```python
from build123d import *

# Parameters (mm, degrees)
BOSS_EXTRUDE1_DEPTH = 40
SKETCH2_R           = 27
CUT_EXTRUDE3_DEPTH  = 10
SKETCH4_R           = 19
CUT_EXTRUDE4_DEPTH  = 10
SKETCH5_R           = 19
BOSS_EXTRUDE2_DEPTH = 20
SKETCH6_R           = 10
CUT_EXTRUDE6_DEPTH  = 20
BOSS_EXTRUDE4_START = 64
SKETCH7_R           = 5
BOSS_EXTRUDE4_DEPTH = 10


with BuildPart() as part:
    # Sketch1 → Boss-Extrude1 (new body)
    with BuildSketch(Plane.XY):
        Polygon((0, 0), (0, 64), (-6, 64), (-6, 69), (3, 100), (73, 100), (82, 69), (82, 64), (76, 64), (76, 0), (56, 0), (56, 20), (20, 20), (20, 0), align=None)
    extrude(amount=BOSS_EXTRUDE1_DEPTH)

    # Sketch2 → Cut-Extrude3 (cut)
    with BuildSketch(Plane.XY.offset(40)):
        with Locations((38, 100)):
            Circle(SKETCH2_R)
    extrude(amount=-CUT_EXTRUDE3_DEPTH, mode=Mode.SUBTRACT)

    # Sketch4 → Cut-Extrude4 (cut)
    with BuildSketch(Plane.XY.offset(30)):
        with Locations((38, 100)):
            Circle(SKETCH4_R)
    extrude(amount=-CUT_EXTRUDE4_DEPTH, mode=Mode.SUBTRACT)

    # Sketch5 → Boss-Extrude2 (add)
    with BuildSketch(Plane.XY.offset(20)):
        with Locations((38, 100)):
            Circle(SKETCH5_R)
    extrude(amount=-BOSS_EXTRUDE2_DEPTH)

    # Sketch6 → Cut-Extrude6 (cut)
    with BuildSketch(Plane.XY.offset(20)):
        with Locations((38, 100)):
            Circle(SKETCH6_R)
    extrude(amount=-CUT_EXTRUDE6_DEPTH, mode=Mode.SUBTRACT)

    # Sketch7 → Boss-Extrude4 (add)
    # profile 1 of 2: a face of its own
    with BuildSketch(Plane(origin=(0, 0, 0), x_dir=(1, 0, 0), z_dir=(0, 1, 0)).offset(BOSS_EXTRUDE4_START)):
        with BuildLine():
            Line((82, -10), (77.667968987, -10))
            Line((77.667968987, -10), (77.667968987, -30))
            Line((77.667968987, -30), (82, -30))
            Line((82, -30), (101, -30))
            ThreePointArc((101, -30), (111, -20), (101, -10))
            Line((101, -10), (82, -10))
        make_face()
        with Locations(Location((101, -20, 0), (0, 0, 90))):
            Circle(SKETCH7_R, mode=Mode.SUBTRACT)
    # profile 2 of 2: a face of its own
    with BuildSketch(Plane(origin=(0, 0, 0), x_dir=(1, 0, 0), z_dir=(0, 1, 0)).offset(BOSS_EXTRUDE4_START)):
        with BuildLine():
            Line((-6, -10), (-2.389922535, -10))
            Line((-2.389922535, -10), (-2.389922535, -30))
            Line((-2.389922535, -30), (-6, -30))
            Line((-6, -30), (-25, -30))
            ThreePointArc((-25, -30), (-35, -20), (-25, -10))
            Line((-25, -10), (-6, -10))
        make_face()
        with Locations(Location((-25, -20, 0), (0, 0, 270))):
            Circle(SKETCH7_R, mode=Mode.SUBTRACT)
    extrude(amount=BOSS_EXTRUDE4_DEPTH)


solid = part.part
```
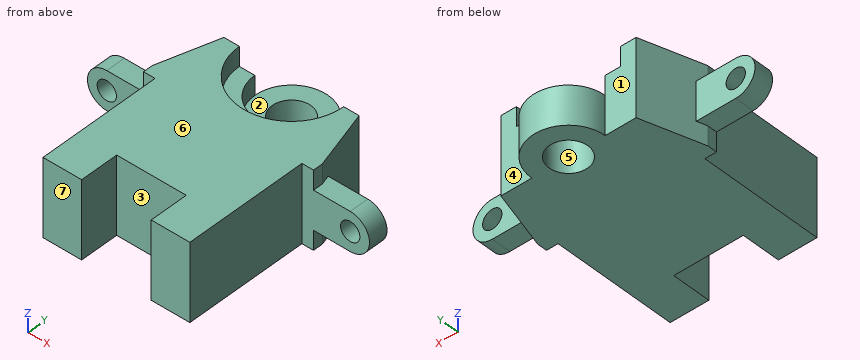
Could you check a few things on this model? Use its own coordinates, in mm. Face numbers are marked on the shaded views. A direction names the side the tool comes from. Coordinates: 2 decimals unless noted, no trailing zeros. Loops run counter-clockwise (first coordinate to the right, second up) from the corner with the lowest first, then second, coordinate; pieces in that order, holes last.
1) Imagine slicing it at A-A (x = 38). List the corners of the cut face in (y, z) for me, and give its area (3 significant figures).
Reported:
outline: (20, 0) - (90, 0) - (90, 20) - (81, 20) - (81, 30) - (73, 30) - (73, 40) - (20, 40) - close; (110, 0) - (119, 0) - (119, 20) - (110, 20) - close
area: 2,720 mm2
2) Thinking about a two-plate mould opening in Y: for the marked faces 5, 6 and 7, which applies, released by +Y, released by -Y, zero draft, split by the parting line, or undercut?
Reported:
face 5: undercut
face 6: zero draft
face 7: released by -Y
3) Which directions (+Z, -Z, +X, -X, +Y, -Y) give clear straight access to the entire face, cutting with the end or side of a thin tool? Please do the marked faces 1, 2, 3 and 4.
Reported:
face 1: +Z, -Z, -X, +Y
face 2: +Z, +Y
face 3: +Z, -Z, -Y
face 4: +Z, -Z, +X, +Y
4) Please list where these lines run through material, in increasing order: line 1 along X through (y, z) = (72, 20); line 2 along X through (y, z) = (18.5, 19); line 3 along Y through (x, z) = (38, 7).
Reported:
line 1: x = -35 to -30, -20 to 96, 106 to 111
line 2: x = 0 to 20, 56 to 76
line 3: y = 20 to 90, 110 to 119
5) Will these pins go through, and if not, where does the flat tip stop? pin 1 Ø10.5 at (x, z) = (86, 19.5) entering from -Y; pin 2 Ø10 at (x, z) = (54.5, 14.5) entering from +Y; pin 3 Ø2 at (x, z) = (9, 22) entering from -Y; pin 4 Ø16 at (x, y) = (38, 100) entering from +Z.
Reported:
pin 1: stops at y = 64
pin 2: stops at y = 115.12
pin 3: stops at y = 0
pin 4: passes through
6) Imagine slicing it at B-B (y = 97.5). List the corners of the cut face in (x, z) for me, and give its area (3 significant figures).
Reported:
outline: (2.27, 0) - (28.32, 0) - (28.32, 20) - (19.17, 20) - (19.17, 30) - (11.12, 30) - (11.12, 40) - (2.27, 40) - close; (47.68, 0) - (73.73, 0) - (73.73, 40) - (64.88, 40) - (64.88, 30) - (56.83, 30) - (56.83, 20) - (47.68, 20) - close
area: 1,560 mm2
7) Imagine slicing it at C-C (x = 91). List the corners of the cut face in (y, z) for me, and give its area (3 significant figures).
Reported:
outline: (64, 10) - (74, 10) - (74, 30) - (64, 30) - close
area: 200 mm2
8) Imagine slicing it at D-D (y = 26.5). List the corners of the cut face in (x, z) for me, and give its area (3 significant figures).
Reported:
outline: (0, 0) - (76, 0) - (76, 40) - (0, 40) - close
area: 3,040 mm2
